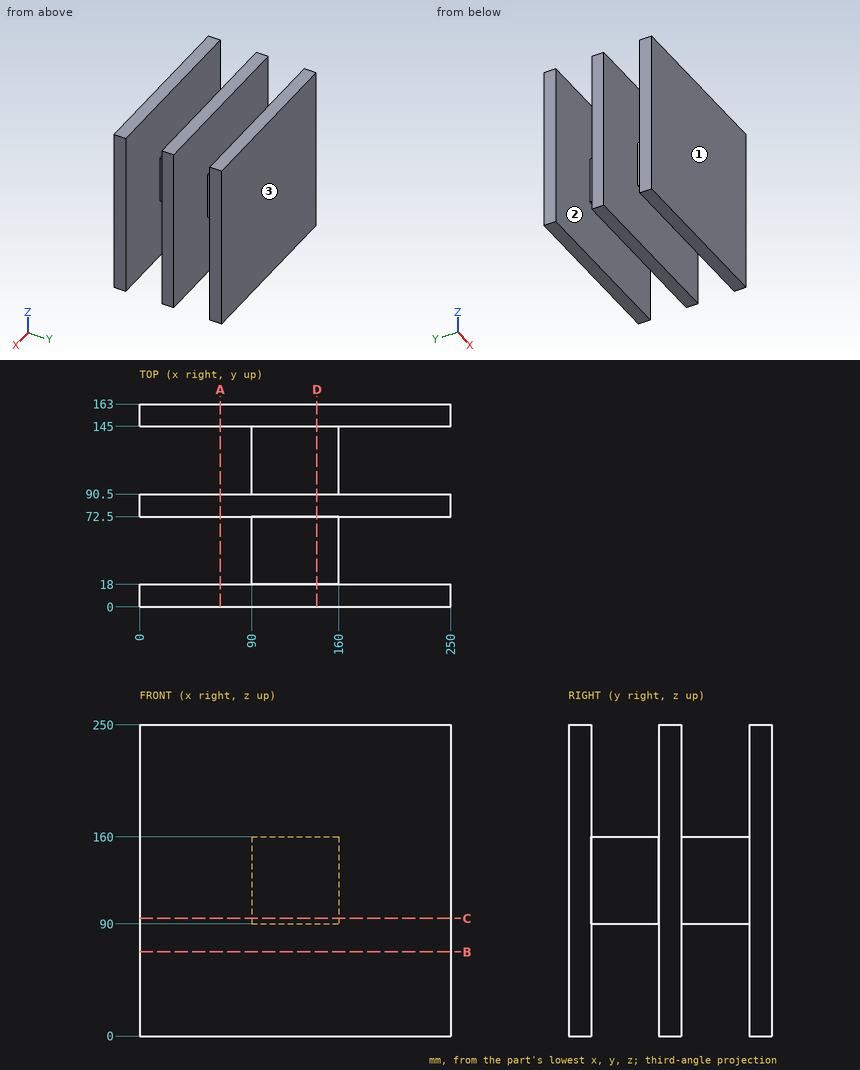
Drawing for the job (mm, zero at the part's lowest x, y, z). Give positions to 0.01 mm unless a question says otherwise; leave off trailing zeros. Write each loop counter-clockwise with the first axis right and the second up, starting at its lowest first coordinate (ties: lowest second). Pieces come first, ordered by that corner, then holes. Notation, with made-up numbers: M -2,15 L 28,15 A27 cw 28,44 Z; hole C 27.5,-13.5 d7. An arc over 180 degrees is marked long. Return JSON: item names as keys, results as strings. Group by question number.
(1) Band-saw the part on B-B (z = 67.5). Give the cut face in (x, y).
(2) Drill centre lines: L1, parallel to Y at x = 79, z = 167.5; L2, parallel to Z at x = 155, y = 99.5. Where is each one in solid material? Low to high. Write a range as [from, to].
(3) Band-saw the part on D-D (x = 142.5). Give the cut face in (y, z), and give its area (3 significant figures).
(4) Band-saw the part on A-A (x = 65). Give the cut face in (y, z), and give its area (3 significant figures).
(5) Mould opens along Y. For the marked faces 1, 2 and 3 say: pulls with the +Y half, pulls with the -Y half, needs draft (parallel to the pull), parting line crosses it, or undercut.
(6) Band-saw the part on C-C (z = 94.5). Give the cut face in (x, y), and give its area (3 significant figures).
(7) Flat gauge pin, fed straight in: pin 1 Ø16.5 at (y, z) = (105.5, 131) entering from -X. Where does the tip first touch, or does it go through?
Entries:
{
 "1": {"outline": "M 0,0 L 250,0 L 250,18 L 0,18 Z; M 0,72.5 L 250,72.5 L 250,90.5 L 0,90.5 Z; M 0,145 L 250,145 L 250,163 L 0,163 Z"},
 "2": {"L1": "y = [0, 18], [72.5, 90.5], [145, 163]", "L2": "z = [90, 160]"},
 "3": {"outline": "M 0,0 L 18,0 L 18,90 L 72.5,90 L 72.5,0 L 90.5,0 L 90.5,90 L 145,90 L 145,0 L 163,0 L 163,250 L 145,250 L 145,160 L 90.5,160 L 90.5,250 L 72.5,250 L 72.5,160 L 18,160 L 18,250 L 0,250 Z", "area": "21,100 mm^2"},
 "4": {"outline": "M 0,0 L 18,0 L 18,250 L 0,250 Z; M 72.5,0 L 90.5,0 L 90.5,250 L 72.5,250 Z; M 145,0 L 163,0 L 163,250 L 145,250 Z", "area": "13,500 mm^2"},
 "5": {"face 1": "pulls with the -Y half", "face 2": "undercut", "face 3": "pulls with the +Y half"},
 "6": {"outline": "M 0,0 L 250,0 L 250,18 L 160,18 L 160,72.5 L 250,72.5 L 250,90.5 L 160,90.5 L 160,145 L 250,145 L 250,163 L 0,163 L 0,145 L 90,145 L 90,90.5 L 0,90.5 L 0,72.5 L 90,72.5 L 90,18 L 0,18 Z", "area": "21,100 mm^2"},
 "7": {"pin 1": "stops at x = 90"}
}
